Can you work these out from the model? Positions are in its coordinate system, mm. A direction names the side the tool comes from. Coordinates: 2 decimals unless noted, no trailing zeros. Loops run counter-clockwise (first coordinate to the right, second up) from the corner with the lowest first, then second, coordinate; pieces in that order, holes last. Notation, with made-up numbers: M -9,-33 L 9,-33 A17 ccw 9,-12 Z; hole C 33.25,-26.5 d3. An arc over 180 degrees is marked long. Answer as a JSON object with one key per item and string values. Group by question number.
Item 1: I'm going to push flat-ended pins straight in: pin 1 Ø8 at (y, z) = (19.5, 94.5) entering from -X; pin 2 Ø5 at (y, z) = (-6, 84.5) entering from +X; pin 3 Ø24 at (x, z) = (-17.5, 75.5) entering from +Y. Where does each tip first touch, or does it pass through?
Item 2: Suppose I cut it at B-B (x = 36). Write out the boundary of the cut face in (y, z), then the cut area to 3 significant figures.
Item 3: We'd pull the mould along X, two halves only. Please class faces 1 (the flat face through (-1, 0, 126)), 2 (the cylindrical face through (-16.752, 12.451, 96.087)), 3 (the flat face through (-67.5, 20, 48)): +X half, -X half, draft (parallel to the pull), parting line (faces both ways), or undercut.
Item 4: Which directions (+Z, -Z, +X, -X, +Y, -Y) give clear straight access to the entire face, cutting with the end or side of a thin tool? Please do faces 4 (the flat face through (19.5, -6, 62)), 5 (the flat face through (-52.5, 40, 51)), 6 (the cylindrical face through (-20.993, 12.451, 81.114)), 7 (the cylindrical face through (-12.57, 12.37, 17.93)), 8 (the flat face through (67.5, 0, 62)).
Item 5: Suppose I cut it at A-A (y = 11.5). Write out the boundary of the cut face in (x, z), then the cut area to 3 significant figures.
Item 6: Suppose I cut it at D-D (x = -56). Write out the boundary of the cut face in (y, z), then the cut area to 3 significant figures.
Item 7: If I drill on line 1 (X direction, y = 61, z = 40.5); line 2 (Y direction, x = 46.5, z = 47); line 3 (X direction, y = 69, z = 41), over which ranges is the centre line in solid material (lowest first)?
Item 8: Suppose I cut it at C-C (z = 106.5). Write out the boundary of the cut face in (x, y).
```python
from build123d import *

# Parameters (mm, degrees)
BOSS_EXTRUDE1_DEPTH      = 126
SKETCH2_R                = 21
SKETCH2_R_2              = 14
BOSS_EXTRUDE4_DEPTH      = 27
BOSS_EXTRUDE4_DEPTH_BACK = 153
BOSS_EXTRUDE5_DEPTH      = 15
BOSS_EXTRUDE7_DEPTH      = 15
BOSS_EXTRUDE8_DEPTH      = 111
SKETCH11_R               = 15
SKETCH11_R_2             = 7.5
BOSS_EXTRUDE9_DEPTH      = 7


with BuildPart() as part:
    # Sketch1 → Boss-Extrude1 (new body)
    with BuildSketch(Plane.XY):
        Polygon((19.5, -9), (19.5, -3), (55.5, -3), (55.5, -9), (67.5, -9), (67.5, 9), (-67.5, 9), (-67.5, -9), align=None)
    extrude(amount=BOSS_EXTRUDE1_DEPTH)



with BuildPart() as body_2:
    # Sketch2 → Boss-Extrude4 (new body, two sides)
    with BuildSketch(Plane.ZY.offset(67.5)) as boss_extrude4_sk:
        with Locations((52.218982883, 87)):
            Circle(SKETCH2_R)
        with Locations((52.218982883, 87)):
            Circle(SKETCH2_R_2, mode=Mode.SUBTRACT)
    extrude(amount=BOSS_EXTRUDE4_DEPTH)
    extrude(boss_extrude4_sk.sketch, amount=-BOSS_EXTRUDE4_DEPTH_BACK)


with BuildPart() as part_1:
    add(part.part)

    add(body_2.part)  # Boss-Extrude5 merges body 2
    # Sketch3 → Boss-Extrude5 (add)
    with BuildSketch(Plane.ZY.offset(67.5)):
        with BuildLine():
            Line((73.218982883, 9), (73.218982883, 87))
            ThreePointArc((73.218982883, 87), (67.068225288, 72.150757595), (52.218982883, 66))
            Line((52.218982883, 66), (38.0233764, 66))
            ThreePointArc((38.0233764, 66), (35.18679718, 65.117501467), (33.351528761, 62.781527332))
            Line((33.351528761, 62.781527332), (16.980511395, 19.850443731))
            ThreePointArc((16.980511395, 19.850443731), (17.86746527, 12.461473248), (24.455467618, 9))
            Line((24.455467618, 9), (73.218982883, 9))
        make_face()
    extrude(amount=-BOSS_EXTRUDE5_DEPTH)

    # Sketch7 → Boss-Extrude7 (add)
    with BuildSketch(Plane.ZY.offset(-43.5)):
        with BuildLine():
            Line((73.218982883, 9), (73.218982883, 87))
            ThreePointArc((73.218982883, 87), (67.068225288, 72.150757595), (52.218982883, 66))
            Line((52.218982883, 66), (38.0233764, 66))
            ThreePointArc((38.0233764, 66), (35.18679718, 65.117501467), (33.351528761, 62.781527332))
            Line((33.351528761, 62.781527332), (16.980511395, 19.850443731))
            ThreePointArc((16.980511395, 19.850443731), (17.86746527, 12.461473248), (24.455467618, 9))
            Line((24.455467618, 9), (73.218982883, 9))
        make_face()
    extrude(amount=BOSS_EXTRUDE7_DEPTH)

    # Sketch4 → Boss-Extrude8 (add)
    with BuildSketch(Plane.ZY.offset(67.5)):
        with BuildLine():
            ThreePointArc((52.218982883, 66), (34.925476722, 75.086367277), (32.597222798, 94.482414795))
            Line((32.597222798, 94.482414795), (0, 9))
            Line((0, 9), (24.455467618, 9))
            ThreePointArc((24.455467618, 9), (17.86746527, 12.461473248), (16.980511395, 19.850443731))
            Line((16.980511395, 19.850443731), (33.351528761, 62.781527332))
            ThreePointArc((33.351528761, 62.781527332), (35.18679718, 65.117501467), (38.0233764, 66))
            Line((38.0233764, 66), (52.218982883, 66))
        make_face()
    extrude(amount=-BOSS_EXTRUDE8_DEPTH)

    # Sketch11 → Boss-Extrude9 (add)
    with BuildSketch(Plane(origin=(0, 9, 0), x_dir=(1, 0, 0), z_dir=(0, 1, 0))):
        with Locations((-13.5, -81.444044499)):
            Circle(SKETCH11_R)
        with Locations((-13.5, -81.444044499)):
            Circle(SKETCH11_R_2, mode=Mode.SUBTRACT)
    extrude(amount=BOSS_EXTRUDE9_DEPTH)


solid = part_1.part
```
From the geometry:
{
 "1": {"pin 1": "x = -23.57", "pin 2": "x = 67.5", "pin 3": "y = 104.71"},
 "2": {"outline": "M -3,0 L 9,0 L 94.48,32.6 A21 ccw 87,73.22 L 9,73.22 L 9,126 L -3,126 Z; hole C 87,52.22 d28", "area": "6,140 mm2"},
 "3": {"face 1": "draft", "face 2": "undercut", "face 3": "-X half"},
 "4": {"face 4": "+Z, -Z, -Y", "face 5": "+Z", "face 6": "+Y", "face 7": "none", "face 8": "+Z, -Z, +X, -Y"},
 "5": {"outline": "M -67.5,0.95 L 43.5,0.95 L 43.5,73.22 L 28.5,73.22 L 28.5,18.65 L -52.5,18.65 L -52.5,73.22 L -67.5,73.22 Z; C -13.5,81.44 d30; hole C -13.5,81.44 d15", "area": "4,130 mm2"},
 "6": {"outline": "M -9,0 L 9,0 L 94.48,32.6 A21 ccw 87,73.22 L 9,73.22 L 9,126 L -9,126 Z; hole C 87,52.22 d28", "area": "6,900 mm2"},
 "7": {"line 1": "-67.5 to -52.5, 28.5 to 43.5", "line 2": "-3 to 9, 66.66 to 74.01, 99.99 to 107.34", "line 3": "-67.5 to 43.5"},
 "8": {"outline": "M -67.5,-9 L 19.5,-9 L 19.5,-3 L 55.5,-3 L 55.5,-9 L 67.5,-9 L 67.5,9 L -67.5,9 Z"}
}
